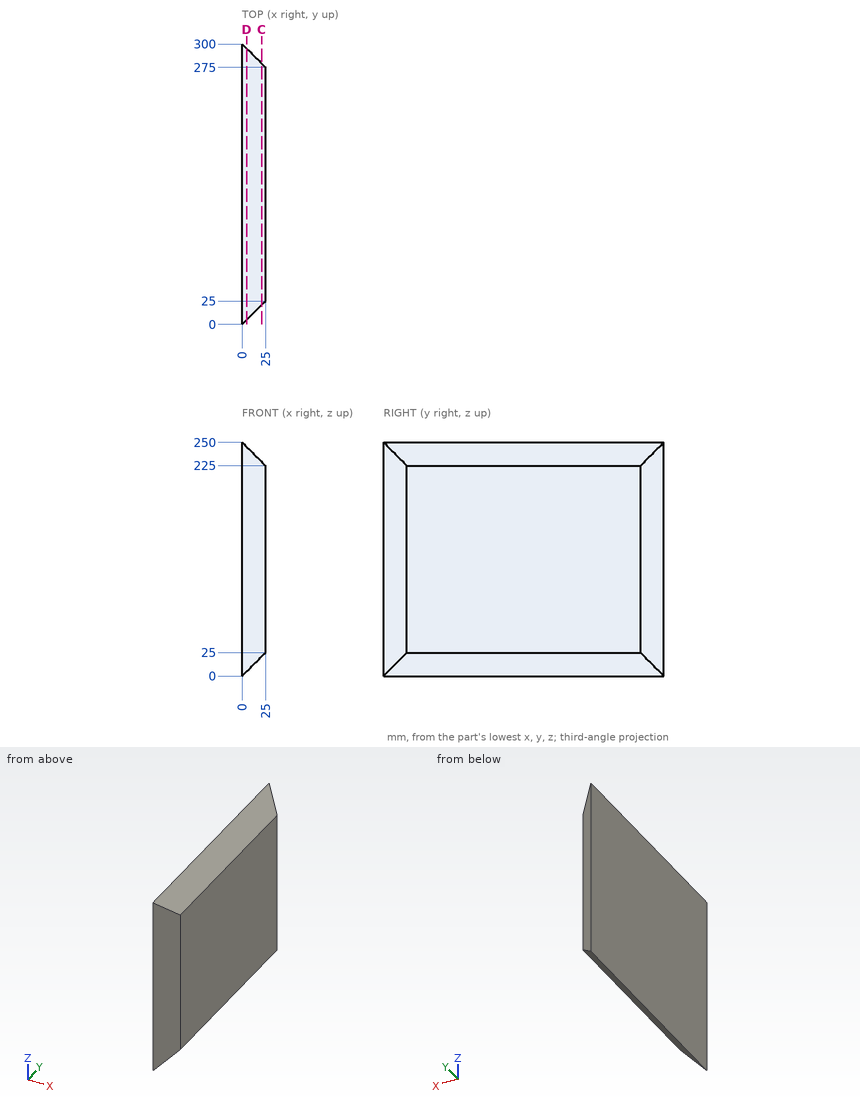
Here's the drawing with two shaded views (mm, measured from the low corner). I have some questions. Give positions to 0.01 mm unless a question says otherwise; leave off trailing zeros. Write each loop counter-clockwise with the first axis right and the second up, starting at its lowest first coordinate (ties: lowest second). Pieces come first, ordered by that corner, then holes. Notation, with made-up numbers: (27, 14) -> (55, 14) arc R15 ccw to (55, 18) -> close; hole circle Ø7 at (-37, 5.5). An arc over 180 degrees is marked (long way). Use one line per item in the form item = value. Start each with the question number.
1. Imagine slicing it at C-C on x = 20.75. List the corners of the cut face in (y, z) for me.
2. Imagine slicing it at D-D on x = 4.75. List the corners of the cut face in (y, z) for me.
3. If I drill on L1, parallel to X at y = 277.5, z = 24; L2, parallel to Y at x = 24.25, z = 92; L3, parallel to Z at x = 8.5, y = 66.5, over which ranges is the centre line in solid material (lowest first)?
4. Will these pins go through, and if not, where does the flat tip stop? pin 1 Ø6 at (x, y) = (13.5, 193) entering from -Z; pin 2 Ø10 at (x, y) = (6.5, 138) entering from -Z; pin 3 Ø8 at (x, y) = (7, 182) entering from +Z.
Entries:
q1.outline = (20.75, 20.75) -> (279.25, 20.75) -> (279.25, 229.25) -> (20.75, 229.25) -> close
q2.outline = (4.75, 4.75) -> (295.25, 4.75) -> (295.25, 245.25) -> (4.75, 245.25) -> close
q3.L1 = 0 to 22.5
q3.L2 = 24.25 to 275.75
q3.L3 = 8.5 to 241.5
q4.pin_1 = 10.5
q4.pin_2 = 1.5
q4.pin_3 = 247
